Read the model definition and answer for the solid it produces. Units are mm, in the model's axes. Face numbers are marked on the shaded views. Give positions to 0.01 mm unless a question says otherwise; leave off trailing zeros. Order: outer loops, then holes, each group sorted by start corner. A loop starts at its lowest first (then second) coordinate and runs counter-clockwise, first axis right, second up. Notation, with made-up numbers: (33.5, 7) -> (70.5, 7) arc R10 ccw to (70.5, 17) -> close; hole circle Ø8 at (0, -22.75). An arc over 180 degrees is marked (long way). One line per question, with ' | ' between items. Start each with the question number.
Autodesk Fusion 360 part; units mm, degrees
sketch "Sketch1" plane through (0, 0, 0) normal (0, 0, 1) x (1, 0, 0)
  circle A0 centre (0, 0) radius 8
  line L0 (0, 0) -> (0, 8) construction
  line L1 (0, 0) -> (-8, 0) construction
  line L2 (0, 0) -> (8, 0) construction
  line L3 (0, 0) -> (0, -8) construction
  line L4 (-4.6188, 8) -> (-9.2376, 0) construction
  line L5 (-9.2376, 0) -> (-4.6188, -8) construction
  line L6 (-4.6188, -8) -> (4.6188, -8) construction
  line L7 (4.6188, -8) -> (9.2376, 0) construction
  line L8 (9.2376, 0) -> (4.6188, 8) construction
  line L9 (4.6188, 8) -> (-4.6188, 8) construction
  line L10 (-7.5056, -13) -> (7.5056, -13)
  line L11 (7.5056, -13) -> (15.0111, 0)
  line L12 (15.0111, 0) -> (7.5056, 13)
  line L13 (7.5056, 13) -> (-7.5056, 13)
  line L14 (-7.5056, 13) -> (-15.0111, 0)
  line L15 (-15.0111, 0) -> (-7.5056, -13)
  dimension "d1" = 16
  dimension "d4" = 5
extrude "Extrude3" add sketch "Sketch1" along normal blind 14 contours A0 | L10 L11 L12 L13 L14 L15
extrude "Extrude4" cut sketch "Sketch1" along normal through all contours A0
fillet "Fillet2" radius 1 12 edges at (0, 13, 14) (0, 13, 0) (11.2583, 6.5, 14) (11.2583, 6.5, 0) (11.2583, -6.5, 14) (11.2583, -6.5, 0) (-11.2583, 6.5, 14) (-11.2583, 6.5, 0) (-11.2583, -6.5, 0) (-11.2583, -6.5, 14) (0, -13, 0) (0, -13, 14)
thread "Thread2"
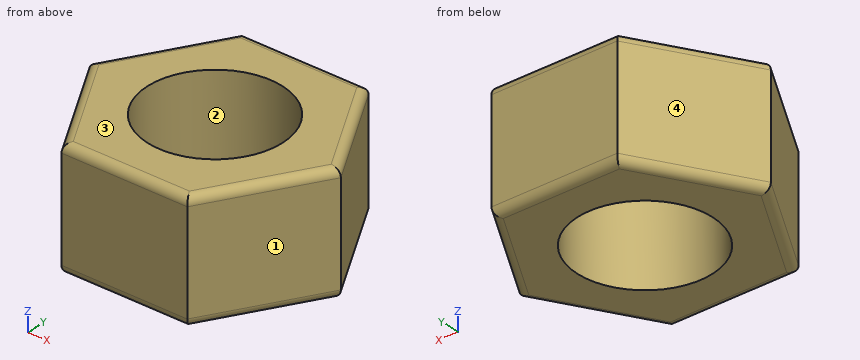
Q1. Determine the mould class of the marked faces 1, 2, 3 and 4 for opening direction X: pulls with the +X half, pulls with the -X half, needs draft (parallel to the pull), parting line crosses it, or undercut.
Q2. A cutting plane is placed at B-B, the plane z = 9.75. Determine the outline of the cut face in (x, y).
Q3. Given P1, Ø2, axis at y = 9.5, z = 9, coming from the -X side; P2, Ø3, axis at y = -1, z = 11.5, coming from the +X side; P3, Ø1.5, axis at x = 11, z = 4.5, coming from the -Y side, each flat-ended and moving along its own axis, determine where each tip first touches the part or whether it passes through.
Q4. A cutting plane is placed at A-A, the plane x = 0. Determine the outline of the cut face in (y, z), then the cut area to 3 significant figures.
Q5. Find the intervals of material crossed by line 1 (Y direction, x = 0, z = 7); line 2 (Y direction, x = 5, z = 12) (3 decimals); line 3 (X direction, y = -5.5, z = 5), in increasing order.
Q6. A cutting plane is placed at C-C, the plane x = -3.5. Determine the outline of the cut face in (y, z), then the cut area to 3 significant figures.
Geometry results:
1) face 1: pulls with the +X half | face 2: undercut | face 3: needs draft | face 4: pulls with the -X half
2) outline: (-15.01, 0) -> (-7.51, -13) -> (7.51, -13) -> (15.01, 0) -> (7.51, 13) -> (-7.51, 13) -> close; hole circle Ø16 at (0, 0)
3) P1: x = -10.1 | P2: x = 15.01 | P3: y = -8.25
4) outline: (-13, 1) arc R1 ccw to (-12, 0) -> (-8, 0) -> (-8, 14) -> (-12, 14) arc R1 ccw to (-13, 13) -> close; (8, 0) -> (12, 0) arc R1 ccw to (13, 1) -> (13, 13) arc R1 ccw to (12, 14) -> (8, 14) -> close | area: 139 mm²
5) line 1: -13 to -8, 8 to 13 | line 2: -13 to -6.245, 6.245 to 13 | line 3: -11.84 to -5.81, 5.81 to 11.84
6) outline: (-13, 1) arc R1 ccw to (-12, 0) -> (-7.19, 0) -> (-7.19, 14) -> (-12, 14) arc R1 ccw to (-13, 13) -> close; (7.19, 0) -> (12, 0) arc R1 ccw to (13, 1) -> (13, 13) arc R1 ccw to (12, 14) -> (7.19, 14) -> close | area: 162 mm²
